Geometry: final body of the model. Coordinates: model frame, mm. Face numbers are marked on the shaded views. A direction names the side the tool comes from. Round coordinates to 2 decimals unless told otherwise and drop trailing zeros. Order: outer loops, then holes, each group sorted by start corner. A loop starts at its lowest first (then second) coordinate and runs counter-clockwise, first axis right, second up. Notation, with made-up numbers: M -4,-5 L 50,-5 A29 cw 50,24 Z; hole C -39,15.5 d8. An arc over 180 degrees is marked long. Put each result on its own line as item: value. Start each with the question number.
1) Section D-D, the plane y = -20. Return loops of the section in (x, z).
2) Section C-C, the plane z = -7. Return loops of the section in (x, y), then the cut area to 3 significant figures.
3) Draft query along Z for the marked faces 1, 2, 3 and 4. Return one class per face: pulls with the +Z half, pulls with the -Z half, needs draft (parallel to the pull), parting line crosses it, or undercut.
4) Access query for the marked faces 5, 6 and 7. Directions: +Z, -Z, +X, -X, +Y, -Y. A direction counts if a zero-diameter tool reaches every point of the face in a straight line with its end or side. Return the directions, or none.
5) Material intervals for probe 1 along Z at (x, y) = (20, -2); probe 2 along Y at (x, z) = (10, -12.5); probe 3 along Z at (x, y) = (-15, -7.5), sorted ascending. Write a range as [from, to].
6) First-contact query: P1, Ø9.5, axis at y = -18.5, z = -4, coming from the +X side; P2, Ø6, axis at x = 17.5, z = -10.5, coming from the +Y side; P3, Ø8, axis at y = -14, z = 8, coming from the -X side. Flat tips, straight axial feed; report the tip coordinate or a pass-through.
7) Section B-B, the plane x = 8.5. Return loops of the section in (y, z).
8) Section A-A, the plane y = -14.25. Return loops of the section in (x, z).
from build123d import *

# Parameters (mm, degrees)
F0_W      = 69.85
F0_H      = 31.75
F1_DEPTH  = 25.4
F3_DEPTH  = 25.4
F4_W      = 40.9290131211
F4_H      = 25.4
F5_DEPTH  = 25.4
F7_DEPTH  = 25.4
F9_DEPTH  = 25.4
F11_DEPTH = 25.4
F12_R     = 5.3255513917
F13_DEPTH = 25.4


with BuildPart() as f1:
    # F0 (on Front) → F1 (new body)
    with BuildSketch(Plane.XZ):
        with Locations((6.0040131211, -2.1042692847)):
            Rectangle(F0_W, F0_H)
    extrude(amount=F1_DEPTH)

    # F2 (on face) → F3 (cut)
    with BuildSketch(Plane.XZ.offset(25.4)):
        with BuildLine():
            ThreePointArc((-28.9209868789, 0), (-25.5531384198, 8.8906260106), (-17.3940813557, 13.7707307153))
            Line((-17.3940813557, 13.7707307153), (-28.9209868789, 13.7707307153))
            Line((-28.9209868789, 13.7707307153), (-28.9209868789, 0))
        make_face()
    extrude(amount=-F3_DEPTH, mode=Mode.SUBTRACT)

    # F4 (on face) → F5 (cut)
    with BuildSketch(Plane.XZ.offset(25.4)):
        with Locations((20.4645065606, 1.0707307153)):
            Rectangle(F4_W, F4_H)
    extrude(amount=-F5_DEPTH, mode=Mode.SUBTRACT)

    # F6 (on face) → F7 (cut)
    with BuildSketch(Plane.XZ.offset(25.4)):
        with BuildLine():
            ThreePointArc((-10.0476886535, 13.7707307153), (-2.7789437741, 8.5233366664), (0, 0))
            Line((0, 0), (0, 13.7707307153))
            Line((0, 13.7707307153), (-10.0476886535, 13.7707307153))
        make_face()
    extrude(amount=-F7_DEPTH, mode=Mode.SUBTRACT)

    # F8 (on face) → F9 (cut)
    with BuildSketch(Plane.XY.offset(-11.6292692847)):
        with BuildLine():
            ThreePointArc((40.9290131211, -15.1913341976), (38.2324702051, -21.3366480861), (32.8915528953, -25.4))
            Line((32.8915528953, -25.4), (40.9290131211, -25.4))
            Line((40.9290131211, -25.4), (40.9290131211, -15.1913341976))
        make_face()
        with BuildLine():
            ThreePointArc((30.6381783403, 0), (37.4598520862, -3.8845668164), (40.9290131211, -10.92658455))
            Line((40.9290131211, -10.92658455), (40.9290131211, 0))
            Line((40.9290131211, 0), (30.6381783403, 0))
        make_face()
    extrude(amount=-F9_DEPTH, mode=Mode.SUBTRACT)

    # F10 (on face) → F11 (cut)
    with BuildSketch(Plane.XY.offset(-11.6292692847)):
        with BuildLine():
            Line((6.9414059162, -19.1323067701), (25.9914059162, -19.1323067701))
            ThreePointArc((25.9914059162, -19.1323067701), (29.9975909424, -14.5264953928), (25.5823172629, -10.3112403303))
            Line((25.5823172629, -10.3112403303), (7.8313201666, -10.3112403303))
            ThreePointArc((7.8313201666, -10.3112403303), (3.3983989935, -14.319447362), (6.9414059162, -19.1323067701))
        make_face()
    extrude(amount=-F11_DEPTH, mode=Mode.SUBTRACT)

    # F12 (on face) → F13 (cut)
    with BuildSketch(Plane.XZ.offset(25.4)):
        with Locations((-14.4604934394, 0)):
            Circle(F12_R)
    extrude(amount=-F13_DEPTH, mode=Mode.SUBTRACT)


solid = f1.part
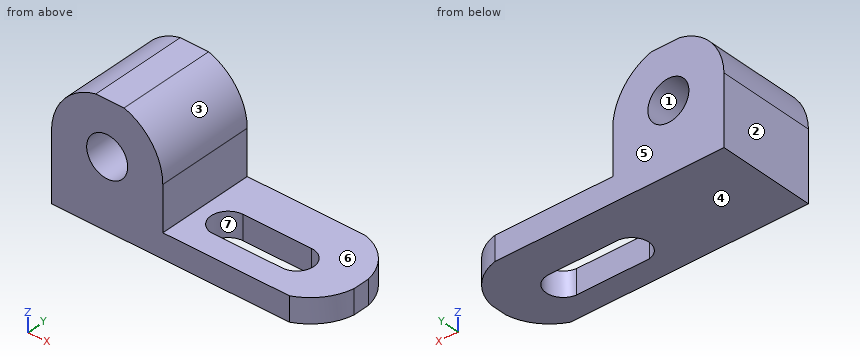
Result sheet:
1. outline: M -28.92,-17.98 L 39.16,-17.98 L 39.16,-11.63 L 0,-11.63 L 0,0 A14.46 ccw -10.05,13.77 L -17.39,13.77 A14.47 ccw -28.92,0 Z; hole C -14.46,0 d10.65
2. outline: M -28.92,-25.4 L 0,-25.4 L 0,0 L -28.92,0 Z
2. area: 735 mm2
3. face 1: undercut
3. face 2: needs draft
3. face 3: pulls with the +Z half
3. face 4: pulls with the -Z half
4. face 5: +Z, -Z, +X, -X, +Y
4. face 6: +Z, +X, +Y, -Y
4. face 7: +Z, -Z
5. probe 1: z = [-17.98, -11.63]
5. probe 2: y = [-25.4, -19.13], [-10.31, 0]
5. probe 3: z = [-17.98, -5.3], [5.3, 13.77]
6. P1: stops at x = 0
6. P2: stops at y = 0
6. P3: stops at x = -28.24
7. outline: M -25.4,-17.98 L -19.13,-17.98 L -19.13,-11.63 L -25.4,-11.63 Z; M -10.31,-17.98 L 0,-17.98 L 0,-11.63 L -10.31,-11.63 Z
8. outline: M -28.92,-17.98 L 3.41,-17.98 L 3.41,-11.63 L 0,-11.63 L 0,0 A14.46 ccw -10.05,13.77 L -17.39,13.77 A14.47 ccw -28.92,0 Z; M 29.98,-17.98 L 40.93,-17.98 L 40.93,-11.63 L 29.98,-11.63 Z; hole C -14.46,0 d10.65
